```python
from build123d import *

# Parameters (mm, degrees)
SKETCH_1_W             = 5
SKETCH_1_H             = 5
EXTRUDE_1_DEPTH        = 8
EXTRUDE_3_DEPTH        = 0.75
FILLET_2_R             = 0.2
FILLET_3_R             = 0.2
SKETCH_5_W             = 4
SKETCH_5_H             = 4
CUT_EXTRUDE_1_DEPTH    = 7
SKETCH_6_W             = 6
SKETCH_6_H             = 0.3
EXTRUDE_4_DEPTH        = 0.6
FILLET_4_R             = 0.1
FILLET_4_OF_MIRROR_1_R = 0.1
FILLET_5_R             = 0.1


# Some blends are built 0.0001 mm under size
with BuildPart() as part:
    # 草图1 → 凸台-拉伸1 (new body)
    with BuildSketch(Plane(origin=(0, 0, 0), x_dir=(0, 0, -1), z_dir=(1, 0, 0))):
        Rectangle(SKETCH_1_W, SKETCH_1_H)
    extrude(amount=EXTRUDE_1_DEPTH)

    # 草图4 → 凸台-拉伸3 (add, symmetric)
    with BuildSketch(Plane(origin=(0, 0, 0), x_dir=(1, 0, 0), z_dir=(0, 1, 0))):
        with BuildLine():
            Line((0, -2.5), (0.530317969, -6.502851582))
            ThreePointArc((0.530317969, -6.502851582), (5.54929459, -9.181591589), (6.474873734, -3.56829687))
            Line((6.474873734, -3.56829687), (5.414213562, -4.628957042))
            ThreePointArc((5.414213562, -4.628957042), (2.779286251, -7.627423723), (5.006963629, -4.315158958))
            Line((5.006963629, -4.315158958), (6.064710581, -2.5))
            Line((6.064710581, -2.5), (0, -2.5))
        make_face()
    extrude(amount=EXTRUDE_3_DEPTH, both=True)

    # 圆角2
    fillet_2_edges = [part.edges().sort_by_distance(p)[0] for p in [
        (5.414213562, 0, 4.628957042),
        (6.474873734, 0, 3.56829687),
    ]]
    fillet(fillet_2_edges, radius=FILLET_2_R)

    # 圆角3
    fillet_3_edges = [part.edges().sort_by_distance(p)[0] for p in [
        (5.006963629, 0, 4.315158958),
    ]]
    fillet(fillet_3_edges, radius=FILLET_3_R)

    # 草图5 → 切除-拉伸1 (cut)
    with BuildSketch(Plane.ZY):
        Rectangle(SKETCH_5_W, SKETCH_5_H)
    extrude(amount=-CUT_EXTRUDE_1_DEPTH, mode=Mode.SUBTRACT)

    # 草图6 → 凸台-拉伸4 (add)
    with BuildSketch(Plane(origin=(0, 2.5, 0), x_dir=(1, 0, 0), z_dir=(0, 1, 0))):
        with Locations((4, 0)):
            Rectangle(SKETCH_6_W, SKETCH_6_H)
        with Locations((4, 1.205749971)):
            Rectangle(SKETCH_6_W, SKETCH_6_H)
        with Locations((4, -1.205749971)):
            Rectangle(SKETCH_6_W, SKETCH_6_H)
    extrude_4 = extrude(amount=-EXTRUDE_4_DEPTH)

    # 圆角4
    fillet_4_edges = [part.edges().sort_by_distance(p)[0] for p in [
        (1, 1.9, 1.205749971),
        (4, 1.9, 1.355749971),
        (4, 1.9, 1.055749971),
        (1, 1.9, 0),
        (4, 1.9, 0.15),
        (4, 1.9, -0.15),
        (1, 1.9, -1.205749971),
        (4, 1.9, -1.055749971),
        (4, 1.9, -1.355749971),
    ]]
    fillet(fillet_4_edges, radius=FILLET_4_R - 0.0001)  # a hair under: the kernel refuses the full size

    # 镜向1: 凸台-拉伸4 across plane
    add(extrude_4.mirror(Plane.ZX))

    # 圆角4 of 镜向1
    fillet_4_of_mirror_1_edges = [part.edges().sort_by_distance(p)[0] for p in [
        (1, -1.9, 1.205749971),
        (4, -1.9, 1.355749971),
        (4, -1.9, 1.055749971),
        (1, -1.9, 0),
        (4, -1.9, 0.15),
        (4, -1.9, -0.15),
        (1, -1.9, -1.205749971),
        (4, -1.9, -1.055749971),
        (4, -1.9, -1.355749971),
    ]]
    fillet(fillet_4_of_mirror_1_edges, radius=FILLET_4_OF_MIRROR_1_R - 0.0001)  # a hair under: the kernel refuses the full size

    # 圆角5
    # the kernel refuses this fillet: 0.1 mm, written as the material it adds along each edge
    with BuildSketch(Plane(origin=(6.314710581, -0.75, 2.5), x_dir=(0, -1, 0), z_dir=(-1, 0, 0))) as fillet_5_piece_1_section:
        with BuildLine():
            CenterArc((FILLET_5_R, FILLET_5_R), FILLET_5_R, 180, 90)
            Line((0, FILLET_5_R), (0, 0))
            Line((0, 0), (FILLET_5_R, 0))
        make_face()
    fillet_5_piece_1 = extrude(amount=6.314710581, mode=Mode.PRIVATE)
    fillet_5_piece_1 = split(fillet_5_piece_1, bisect_by=Plane(origin=(0.055159567, -0.772671932, 2.916345616), z_dir=(0.9913377232664815, 0, -0.1313374220427252)), keep=Keep.TOP, mode=Mode.PRIVATE)
    fillet_5_piece_1 = split(fillet_5_piece_1, bisect_by=Plane(origin=(5.284914857, -0.772671932, 3.83817752), z_dir=(-0.8640058232036738, 0, -0.5034818144383589)), keep=Keep.TOP, mode=Mode.PRIVATE)
    add(fillet_5_piece_1)
    with BuildSketch(Plane(origin=(6.064710581, 0.75, 2.5), x_dir=(1, 0, 0), z_dir=(0, -1, 0))) as fillet_5_piece_2:
        with BuildLine():
            CenterArc((FILLET_5_R * 0.57466995271, FILLET_5_R), FILLET_5_R, 210.230623586, 59.769376414)
            Line((-FILLET_5_R * 0.289335870494, FILLET_5_R * 0.496518185562), (0, 0))
            Line((0, 0), (FILLET_5_R * 0.57466995271, 0))
        make_face()
    extrude(amount=1.5)
    with BuildSketch(Plane(origin=(6.314710581, 0.75, 2.5), x_dir=(0, 1, 0), z_dir=(-1, 0, 0))) as fillet_5_piece_3_section:
        with BuildLine():
            CenterArc((FILLET_5_R, -FILLET_5_R), FILLET_5_R, 90, 90)
            Line((0, -FILLET_5_R), (0, 0))
            Line((0, 0), (FILLET_5_R, 0))
        make_face()
    fillet_5_piece_3 = extrude(amount=6.314710581, mode=Mode.PRIVATE)
    fillet_5_piece_3 = split(fillet_5_piece_3, bisect_by=Plane(origin=(0.055159567, 0.772671932, 2.916345616), z_dir=(0.9913377232664815, 0, -0.1313374220427252)), keep=Keep.TOP, mode=Mode.PRIVATE)
    fillet_5_piece_3 = split(fillet_5_piece_3, bisect_by=Plane(origin=(5.284914857, 0.772671932, 3.83817752), z_dir=(-0.8640058232036738, 0, -0.5034818144383589)), keep=Keep.TOP, mode=Mode.PRIVATE)
    add(fillet_5_piece_3)
    with BuildSketch(Plane(origin=(6.064710581, 0.75, 2.5), x_dir=(1, 0, 0), z_dir=(0, -1, 0))) as fillet_5_piece_4a_section:
        with BuildLine():
            CenterArc((FILLET_5_R * 0.57466995271, FILLET_5_R), FILLET_5_R, 210.230623586, 59.769376414)
            Line((-FILLET_5_R * 0.289335870494, FILLET_5_R * 0.496518185562), (0, 0))
            Line((0, 0), (FILLET_5_R * 0.57466995271, 0))
        make_face()
    fillet_5_piece_4a = extrude(amount=1.643667488, mode=Mode.PRIVATE)
    fillet_5_piece_4a = split(fillet_5_piece_4a, bisect_by=Plane(origin=(6.070891015, -0.75, 2.510754755), z_dir=(0, -1, 0)), keep=Keep.TOP, mode=Mode.PRIVATE)
    with BuildSketch(Plane(origin=(6.314710581, -0.75, 2.5), x_dir=(0, -1, 0), z_dir=(-1, 0, 0))) as fillet_5_piece_4b_section:
        with BuildLine():
            CenterArc((FILLET_5_R, FILLET_5_R), FILLET_5_R, 180, 90)
            Line((0, FILLET_5_R), (0, 0))
            Line((0, 0), (FILLET_5_R, 0))
        make_face()
    fillet_5_piece_4b = extrude(amount=6.314710581, mode=Mode.PRIVATE)
    fillet_5_piece_4b = split(fillet_5_piece_4b, bisect_by=Plane(origin=(6.084353102, -0.772031599, 2.466292222), z_dir=(0.8640058232036738, 0, 0.5034818144383589)), keep=Keep.TOP, mode=Mode.PRIVATE)
    fillet_5_piece_4 = fillet_5_piece_4a & fillet_5_piece_4b
    add(fillet_5_piece_4)
    with BuildSketch(Plane(origin=(6.314710581, 0.75, 2.5), x_dir=(0, 1, 0), z_dir=(-1, 0, 0))) as fillet_5_piece_5a_section:
        with BuildLine():
            CenterArc((FILLET_5_R, -FILLET_5_R), FILLET_5_R, 90, 90)
            Line((0, -FILLET_5_R), (0, 0))
            Line((0, 0), (FILLET_5_R, 0))
        make_face()
    fillet_5_piece_5a = extrude(amount=6.314710581, mode=Mode.PRIVATE)
    fillet_5_piece_5a = split(fillet_5_piece_5a, bisect_by=Plane(origin=(6.084353102, 0.772031599, 2.466292222), z_dir=(0.8640058232036738, 0, 0.5034818144383589)), keep=Keep.TOP, mode=Mode.PRIVATE)
    with BuildSketch(Plane(origin=(6.064710581, 0.893667488, 2.5), x_dir=(1, 0, 0), z_dir=(0, -1, 0))) as fillet_5_piece_5b_section:
        with BuildLine():
            CenterArc((FILLET_5_R * 0.57466995271, FILLET_5_R), FILLET_5_R, 210.230623586, 59.769376414)
            Line((-FILLET_5_R * 0.289335870494, FILLET_5_R * 0.496518185562), (0, 0))
            Line((0, 0), (FILLET_5_R * 0.57466995271, 0))
        make_face()
    fillet_5_piece_5b = extrude(amount=1.643667488, mode=Mode.PRIVATE)
    fillet_5_piece_5b = split(fillet_5_piece_5b, bisect_by=Plane(origin=(6.070891015, 0.75, 2.510754755), z_dir=(0, 1, 0)), keep=Keep.TOP, mode=Mode.PRIVATE)
    fillet_5_piece_5 = fillet_5_piece_5a & fillet_5_piece_5b
    add(fillet_5_piece_5)


solid = part.part
```
Model file for the job. Use its own axes, mm. A direction names the side the tool comes from. Coordinates: 2 decimals unless noted, no trailing zeros. Order: outer loops, then holes, each group sorted by start corner. A loop starts at its lowest first (then second) coordinate and runs counter-clockwise, first axis right, second up. Notation, with made-up numbers: (-23.75, 60.5) -> (4.25, 60.5) arc R26 ccw to (4.25, 80.5) -> close; hole circle Ø3 at (34, 14). An arc over 180 degrees is marked (long way). Return JSON: item names as keys, results as strings.
Item 1: Slice it at A-A (y = 1.7). Write the cut outline in (x, z), then the cut area to 3 significant figures.
Model answer:
{"outline": "(0, -2.5) -> (8, -2.5) -> (8, 2.5) -> (0, 2.5) -> (0, 2) -> (7, 2) -> (7, -2) -> (0, -2) -> close", "area": "12.0 mm²"}
Item 2: Slice it at C-C (x = 4). Count the separate pieces of the cut face and the enclosed holes in it, then the cut area to 3 significant figures.
Model answer:
{"separate pieces": "2", "enclosed holes": "1", "area": "13.7 mm²"}
Item 3: 3-axis set-ups, long thin cutter, end or side, ignore diameter. For faces 4 (the face through (8, 0, 0)), 5 (the face through (4, 2.5, 0)), 6 (the face through (3, 0, -2)), 7 (the face through (2, -0.75, 5)), 8 (the face through (2, 0.75, 7)): which of +Z, -Z, +X, -X, +Y, -Y reach the whole face in a straight line?
Model answer:
{"face 4": "+Z, -Z, +X, +Y, -Y", "face 5": "+Z, -Z, +X, -X, +Y", "face 6": "-X", "face 7": "+Z, +X, -X, -Y", "face 8": "+Z, +X, -X, +Y"}
Item 4: Mould opens along Z. For faces 1 (the face through (4, 0, -2.5)), 2 (the face through (0, 0, 2.3)), 3 (the face through (3, 0, 2)) say: pulls with the +Z half, pulls with the -Z half, needs draft (parallel to the pull), parting line crosses it, or undercut.
Model answer:
{"face 1": "pulls with the -Z half", "face 2": "needs draft", "face 3": "undercut"}
Item 5: Wall check: line 1 along Z through (x, y) = (4, -0.35); line 2 along Y through (x, z) = (6.75, -1.25); line 3 along Z through (x, y) = (4.5, -0.15). Give the ranges that are in metal, low to high. Write a range as from..to.
Model answer:
{"line 1": "z = -2.5..-2, 2..4.04, 8.04..9.54", "line 2": "y = -2.5..-1.9, 1.9..2.5", "line 3": "z = -2.5..-2, 2..4.11, 7.98..9.51"}
Item 6: Slice it at B-B (z = 7.5). Write the cut outline in (x, y).
Model answer:
{"outline": "(0.82, -0.75) -> (2.63, -0.75) -> (2.63, 0.75) -> (0.82, 0.75) -> close; (5.37, -0.75) -> (7.18, -0.75) -> (7.18, 0.75) -> (5.37, 0.75) -> close"}
Item 7: Pin check, flat tips, straight feed: P1, Ø2.5, axis at x = 4.5, y = 0, coming from the +Z side; P2, Ø3.5, axis at x = 2.5, z = 6, coming from the -Y side. Stop position of each tip, or through.
Model answer:
{"P1": "stops at z = 9.54", "P2": "stops at y = -0.75"}
